The model under review builds one solid part; all positions refer to its coordinate system, in mm. Face numbers are marked on the shaded views. A direction names the side the tool comes from. Coordinates: 2 decimals unless noted, no trailing zeros. Order: outer loops, then holes, each group sorted by start corner. A loop starts at its lowest first (then second) coordinate and runs counter-clockwise, first axis right, second up. Notation, with made-up numbers: (35, 87) - (43, 87) arc R8 ccw to (43, 91) - close; hole circle Ø5 at (-14.5, 74). An arc over 180 degrees is marked (long way). Answer in a Markdown table with one row per item.
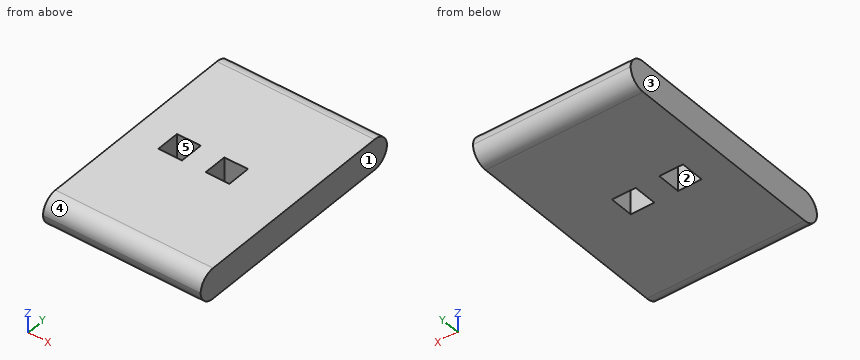
Autodesk Inventor part; units mm, degrees
sketch "Skizze1" plane through (0, 0, 0) normal (0, 0, 1) x (1, 0, 0)
  line L0 (-5, 7.5) -> (5, 7.5)
  line L1 (5, 7.5) -> (5, -7.5)
  line L2 (5, -7.5) -> (-5, -7.5)
  line L3 (-5, -7.5) -> (-5, 7.5)
  line L4 (-7, 0) -> (7, 0)
  line L5 (0, 10.5) -> (0, -10.5)
  point P0 (0, 0)
  dimension "d0" = 10
  dimension "d1" = 15
extrude "Extrusion1" add sketch "Skizze1" along normal mid plane 1.95
sketch "Skizze2" plane through (0, 0, 0.975) normal (0, 0, 1) x (1, 0, 0)
  line L0 (-5, 7.5) -> (-5, -7.5)
  line L1 (-3, -0.75) -> (-1.5, -0.75)
  line L2 (-1.5, -0.75) -> (-1.5, 0.75)
  line L3 (-1.5, 0.75) -> (-3, 0.75)
  line L4 (-3, 0.75) -> (-3, -0.75)
  line L5 (0, -0.75) -> (1.5, -0.75)
  line L6 (1.5, -0.75) -> (1.5, 0.75)
  line L7 (1.5, 0.75) -> (0, 0.75)
  line L8 (0, 0.75) -> (0, -0.75)
  line L9 (-7, 0) -> (7, 0)
  point P0 (0, 0)
  dimension "d4" = 1.5
  dimension "d5" = 2
  dimension "d6" = 1.5
  dimension "d7" = 1.5
  dimension "d8" = 1.5
extrude "Extrusion2" cut sketch "Skizze2" against normal blind 1.95
fillet "Rundung1" radius 1 4 edges at (0, 7.5, 0.975) (0, 7.5, -0.975) (0, -7.5, -0.975) (0, -7.5, 0.975)
properties part number "ChassisRechtsUntenKlappeSchluessel"
Item 1: To check wall thickness, follow line 1 (X direction, y = -0.5, z = -0.7); line 2 (Y direction, x = -2.5, z = 0.35); line 3 (Y direction, x = -0.75, z = -0.4). State the ranges of each line that lie inside material, in increasing order. Write a range as from..to.
Check values:
| item | result |
|---|---|
| line 1 | -5..-3, -1.5..0, 1.5..5 |
| line 2 | -7.43..-0.75, 0.75..7.43 |
| line 3 | -7.41..7.41 |
Item 2: We need section B-B, the plane y = -0.5. Write out the cut boundary in (x, z) (3 decimals).
Check values:
| item | result |
|---|---|
| outline | (-5, -0.975) - (-3, -0.975) - (-3, 0.975) - (-5, 0.975) - close; (-1.5, -0.975) - (0, -0.975) - (0, 0.975) - (-1.5, 0.975) - close; (1.5, -0.975) - (5, -0.975) - (5, 0.975) - (1.5, 0.975) - close |
Item 3: We need section D-D, the plane z = -0.8. Write out the cut boundary in (x, y).
Check values:
| item | result |
|---|---|
| outline | (-5, -7.07) - (5, -7.07) - (5, 7.07) - (-5, 7.07) - close; hole (-3, -0.75) - (-1.5, -0.75) - (-1.5, 0.75) - (-3, 0.75) - close; hole (0, -0.75) - (1.5, -0.75) - (1.5, 0.75) - (0, 0.75) - close |
Item 4: Mouldability with a two-part tool opening along Y and no side actions: class the marked faces 3, 4 and 5 as +Y half, -Y half, draft (parallel to the pull), parting line (faces both ways), or undercut.
Check values:
| item | result |
|---|---|
| face 3 | draft |
| face 4 | -Y half |
| face 5 | undercut |
Item 5: Tool access review of the marked faces 1 and 2: name each direction out of +Z, -Z, +X, -X, +Y, -Y from which nothing blocks a thin tool from reaching the whole face with its end or side.
Check values:
| item | result |
|---|---|
| face 1 | +Z, -Z, +X, +Y, -Y |
| face 2 | +Z, -Z |
Item 6: We need section A-A, the plane x = -1.75. Write out the cut boundary in (y, z) (3 decimals), then the cut area to 3 significant figures.
Check values:
| item | result |
|---|---|
| outline | (-7.5, 0) arc R1 ccw to (-6.5, -0.975) - (-0.75, -0.975) - (-0.75, 0.975) - (-6.5, 0.975) arc R1 ccw to start; (0.75, -0.975) - (6.5, -0.975) arc R1 ccw to (7.5, 0) arc R1 ccw to (6.5, 0.975) - (0.75, 0.975) - close |
| area | 25.5 mm^2 |
Item 7: Clearance check with a flat-ended pin moving along its axis: pin 1 Ø5 at (x, y) = (-2.5, -0.5) entering from -Z (3 decimals). State where the tip first meets the part, or that it passes through.
Check values:
| item | result |
|---|---|
| pin 1 | z = -0.975 |
Item 8: We need section C-C, the plane z = 0.5. Write out the cut boundary in (x, y), then the cut area to 3 significant figures.
Check values:
| item | result |
|---|---|
| outline | (-5, -7.35) - (5, -7.35) - (5, 7.35) - (-5, 7.35) - close; hole (-3, -0.75) - (-1.5, -0.75) - (-1.5, 0.75) - (-3, 0.75) - close; hole (0, -0.75) - (1.5, -0.75) - (1.5, 0.75) - (0, 0.75) - close |
| area | 143 mm^2 |
